from build123d import *

# Parameters (mm, degrees)
SKETCH1_R           = 98.425
SKETCH1_R_2         = 79.375
BOSS_EXTRUDE1_DEPTH = 6.35
BOSS_EXTRUDE2_START = 6.35
SKETCH2_R           = 9.525
BOSS_EXTRUDE2_DEPTH = 15.24
CIRPATTERN2_COUNT   = 4


with BuildPart() as part:
    # Sketch1 → Boss-Extrude1 (new body)
    with BuildSketch(Plane(origin=(0, 0, 0), x_dir=(0, 0, -1), z_dir=(1, 0, 0))):
        Circle(SKETCH1_R)
        Circle(SKETCH1_R_2, mode=Mode.SUBTRACT)
    extrude(amount=BOSS_EXTRUDE1_DEPTH)

    # Sketch2 → Boss-Extrude2 (add)
    with BuildSketch(Plane(origin=(0, 0, 0), x_dir=(0, 0, -1), z_dir=(1, 0, 0)).offset(BOSS_EXTRUDE2_START)):
        with Locations((88.9, 0)):
            Circle(SKETCH2_R)
    boss_extrude2 = extrude(amount=BOSS_EXTRUDE2_DEPTH)

    # Sketch4 → 1/4 (0.2500) Dowel Hole1 (revolve, cut)
    with BuildSketch(Plane(origin=(21.59, 0, -88.9), x_dir=(0, 0, -1), z_dir=(0, 1, 0))):
        Polygon((0, 0), (0, 14.607732465), (3.175, 12.7), (3.175, 0), align=None)
    f_1_4_0_2500_dowel_hole1 = revolve(axis=Axis((27.94, 0, -88.9), (-1, 0, 0)), mode=Mode.SUBTRACT)

    # CirPattern2: Boss-Extrude2, 1/4 (0.2500) Dowel Hole1 ×4 about axis
    cirpattern2_axis = Axis((0, 0, 0), (1, 0, 0))
    for i in range(1, CIRPATTERN2_COUNT):
        add(boss_extrude2.rotate(cirpattern2_axis, i * 360 / CIRPATTERN2_COUNT))
        add(f_1_4_0_2500_dowel_hole1.rotate(cirpattern2_axis, i * 360 / CIRPATTERN2_COUNT), mode=Mode.SUBTRACT)


solid = part.part
Input: part model. Units: mm. Frame: model coordinates. A direction names the side the tool comes from. Round coordinates to 2 decimals unless told otherwise and drop trailing zeros. Order: outer loops, then holes, each group sorted by start corner. A loop starts at its lowest first (then second) coordinate and runs counter-clockwise, first axis right, second up. Notation, with made-up numbers: (35.25, 88) - (57.25, 88) arc R28 ccw to (57.25, 109) - close; hole circle Ø6 at (45, -33.75). An arc over 180 degrees is marked (long way). Answer as a JSON object with one key per item and string values. Group by question number.
(1) Cut plane C-C (z = 26). Return loops of the section in (x, y), then the cut area to 3 significant figures.
(2) Material intervals for probe 1 along Y at (x, z) = (5, 0) (3 decimals); probe 2 along Y at (x, z) = (17.5, 88.9) (3 decimals), sorted ascending. Write a range as from..to.
(3) Cut plane B-B (y = 21). Return loops of the section in (x, z).
(4) Cut plane A-A (x = 12.5). Return loops of the section in (y, z) (3 decimals), then the cut area to 3 significant figures.
(5) Reachability of faces 1 (the face through (21.59, 4, 89)), 2 (the face through (13.863, -79.384, -0.419)) from +Z, -Z, +X, -X, +Y, -Y: full face, straight path, thin tool, end or side. Return the list, or none.
(6) Draft query along Z for faces 3 (the face through (21.59, 89, -4)), 4 (the face through (7.314, 88.349, -0.024)), 5 (the face through (15.33, 86.38, 1.93)), 6 (the face through (13.863, 79.384, 0.419)). Return one class per face: released by +Z, released by -Z, zero draft, split by the parting line, or undercut.
(7) Pin query (flat end, axial travel): P1, Ø3, axis at y = -60.5, z = -48, coming from the +X side; P2, Ø5, axis at x = 8, y = 19.5, coming from the +Z side; P3, Ø5, axis at x = 8, y = -15, coming from the +Z side; P4, Ø10, axis at x = 5, y = 10.5, coming from the +Z side. Return the tip coordinate at first contact, or that it passes through.
Here are the results:
{
 "1": {"outline": "(0, -94.93) - (6.35, -94.93) - (6.35, -75) - (0, -75) - close; (0, 75) - (6.35, 75) - (6.35, 94.93) - (0, 94.93) - close", "area": "253 mm^2"},
 "2": {"probe 1": "y = -98.425..-79.375, 79.375..98.425", "probe 2": "y = -9.525..-3.175, 3.175..9.525"},
 "3": {"outline": "(0, -96.16) - (6.35, -96.16) - (6.35, -76.55) - (0, -76.55) - close; (0, 76.55) - (6.35, 76.55) - (6.35, 96.16) - (0, 96.16) - close"},
 "4": {"outline": "circle Ø19.05 at (-88.9, 0); circle Ø19.05 at (0, -88.9); circle Ø19.05 at (0, 88.9); circle Ø19.05 at (88.9, 0); hole circle Ø6.35 at (-88.9, 0); hole circle Ø6.35 at (0, -88.9); hole circle Ø6.35 at (0, 88.9); hole circle Ø6.35 at (88.9, 0)", "area": "1,010 mm^2"},
 "5": {"face 1": "+Z, -Z, +X, +Y, -Y", "face 2": "+X"},
 "6": {"face 3": "zero draft", "face 4": "undercut", "face 5": "undercut", "face 6": "split by the parting line"},
 "7": {"P1": "passes through", "P2": "stops at z = 96.83", "P3": "stops at z = 97.55", "P4": "stops at z = 98.27"}
}
